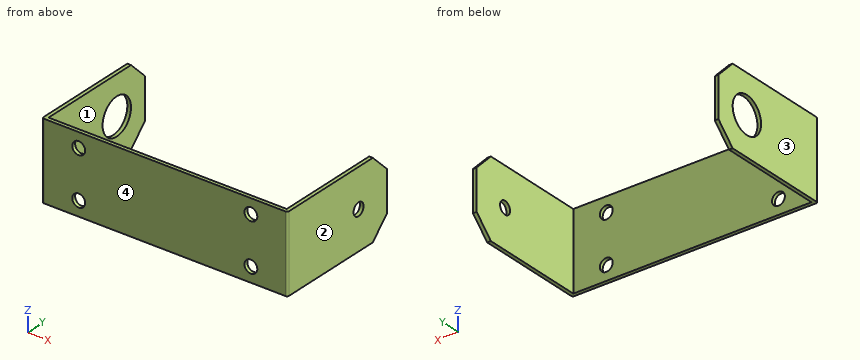
```python
from build123d import *

# Parameters (mm, degrees)
SKETCH_1_W                  = 67
SKETCH_1_H                  = 21
EXTRUDE_1_DEPTH             = 35
SHELL_1_T                   = -1
FILLET_2_R                  = 0.5
CHAMFER_1_SIZE              = 5
HOLE_WIZARD_3_5_3_5_1_D     = 3.5
HOLE_WIZARD_10_0_10_1_D     = 10
HOLE_WIZARD_10_0_10_1_DEPTH = 1
HOLE_WIZARD_3_5_3_5_2_D     = 3.5


with BuildPart() as part:
    # 草图1 → 凸台-拉伸1 (new body)
    with BuildSketch(Plane(origin=(0, 0, 0), x_dir=(1, 0, 0), z_dir=(0, 1, 0))):
        with Locations((-33.5, 10.5)):
            Rectangle(SKETCH_1_W, SKETCH_1_H)
    extrude(amount=EXTRUDE_1_DEPTH)

    # 抽壳1
    shell_1_openings = [part.faces().sort_by_distance(p)[0] for p in [
        (-33.5, 35, -10.5),
        (-33.5, 17.5, 0),
        (-33.5, 17.5, -21),
    ]]
    offset(amount=SHELL_1_T, openings=shell_1_openings, kind=Kind.INTERSECTION)

    # 圆角2
    fillet_2_edges = [part.edges().sort_by_distance(p)[0] for p in [
        (-67, 0, -10.5),
        (0, 0, -10.5),
    ]]
    fillet(fillet_2_edges, radius=FILLET_2_R)

    # 倒角1
    chamfer_1_edges = [part.edges().sort_by_distance(p)[0] for p in [
        (-66.5, 35, 0),
        (-66.5, 35, -21),
        (-0.5, 35, 0),
        (-0.5, 35, -21),
    ]]
    chamfer(chamfer_1_edges, length=CHAMFER_1_SIZE)

    # Ø3.5 (3.5) 直径槽口1 (through all)
    with Locations(Plane(origin=(0, 1, 0), x_dir=(1, 0, 0), z_dir=(0, 1, 0))):
        with Locations((-57, 17), (-10, 17), (-10, 4), (-57, 4)):
            Hole(HOLE_WIZARD_3_5_3_5_1_D / 2)

    # Ø10.0 (10) 直径槽口1
    with Locations(Plane.ZY.offset(67)):
        with Locations((-10.5, 25)):
            Hole(HOLE_WIZARD_10_0_10_1_D / 2, depth=HOLE_WIZARD_10_0_10_1_DEPTH)

    # Ø3.5 (3.5) 直径槽口2 (through all)
    with Locations(Plane(origin=(0, 0, 0), x_dir=(0, 0, -1), z_dir=(1, 0, 0))):
        with Locations((10.5, 25)):
            Hole(HOLE_WIZARD_3_5_3_5_2_D / 2)


solid = part.part
```
Source: CAD feature listing. Evaluate the final solid. Frame: model axes, mm. Face numbers are marked on the shaded views. Coordinates: 2 decimals unless noted, no trailing zeros. Loops run counter-clockwise (first coordinate to the right, second up) from the corner with the lowest first, then second, coordinate; pieces in that order, holes last. Notation, with made-up numbers: (78.5, 21) - (120.5, 21) arc R20 cw to (120.5, 44) - close; hole circle Ø3 at (19.25, 45.5). An arc over 180 degrees is marked (long way). Answer as CSV lines item,"result".
1. Contact query for a flat-ended pin moving along its axis: pin 1 (12 mm diameter, centred on x = -21, z = -11.5, fed in from +Y). Output: stop coordinate, or through.
Established:
pin 1,"stops at y = 1"
2. Section B-B (y = 25). Return loops of the section in (x, z), then the cut area to 3 significant figures.
Established:
outline,"(-67, -21) - (-66, -21) - (-66, -15.5) - (-67, -15.5) - close; (-67, -5.5) - (-66, -5.5) - (-66, 0) - (-67, 0) - close; (-1, -21) - (0, -21) - (0, -12.25) - (-1, -12.25) - close; (-1, -8.75) - (0, -8.75) - (0, 0) - (-1, 0) - close"
area,"28.5 mm2"
3. Mould query, pull axis X, two halves, no side actions, for the marked faces 1, 2, 3 and 4. Classes: released by +X, released by -X, zero draft, split by the parting line, or undercut.
Established:
face 1,"undercut"
face 2,"released by +X"
face 3,"released by -X"
face 4,"zero draft"
4. Section A-A (z = -10.5). Return loops of the section in (x, y).
Established:
outline,"(-67, 0.5) arc R0.5 ccw to (-66.5, 0) - (-0.5, 0) arc R0.5 ccw to (0, 0.5) - (0, 23.25) - (-1, 23.25) - (-1, 1) - (-66, 1) - (-66, 20) - (-67, 20) - close; (-67, 30) - (-66, 30) - (-66, 35) - (-67, 35) - close; (-1, 26.75) - (0, 26.75) - (0, 35) - (-1, 35) - close"
5. Section D-D (y = 9). Return loops of the section in (x, z), then the cut area to 3 significant figures.
Established:
outline,"(-67, -21) - (-66, -21) - (-66, 0) - (-67, 0) - close; (-1, -21) - (0, -21) - (0, 0) - (-1, 0) - close"
area,"42.0 mm2"
6. Ray query, line 1 (Z direction, x = -10, y = 0.65); line 2 (X direction, y = 0.45, z = -17); line 3 (Y direction, x = -66.4, z = -10.5). Return the intervals inside material, ascending.
Established:
line 1,"z = -21 to -18.75, -15.25 to -5.75, -2.25 to 0"
line 2,"x = -67 to -58.75, -55.25 to -11.75, -8.25 to 0"
line 3,"y = 0 to 20, 30 to 35"
7. Section C-C (x = -57). Return loops of the section in (y, z).
Established:
outline,"(0, -21) - (1, -21) - (1, -18.75) - (0, -18.75) - close; (0, -15.25) - (1, -15.25) - (1, -5.75) - (0, -5.75) - close; (0, -2.25) - (1, -2.25) - (1, 0) - (0, 0) - close"
